Design review of the part shown in the three views and the two pictorial views. Dimensions are in mm from the part's minimum x, y and z. A direction names the side the tool comes from. Give positions to 0.01 mm unless a question says otherwise; leave off trailing zeros. Order: outer loops, then holes, each group sorted by start corner. A loop starts at its lowest first (then second) coordinate and runs counter-clockwise, first axis right, second up. Notation, with made-up numbers: (11, -29.5) - (20, -29.5) arc R20 cw to (20, 6.5) - close; hole circle Ø8 at (-9, 74). An arc over 180 degrees is marked (long way). Put each result on its own line as item: value.
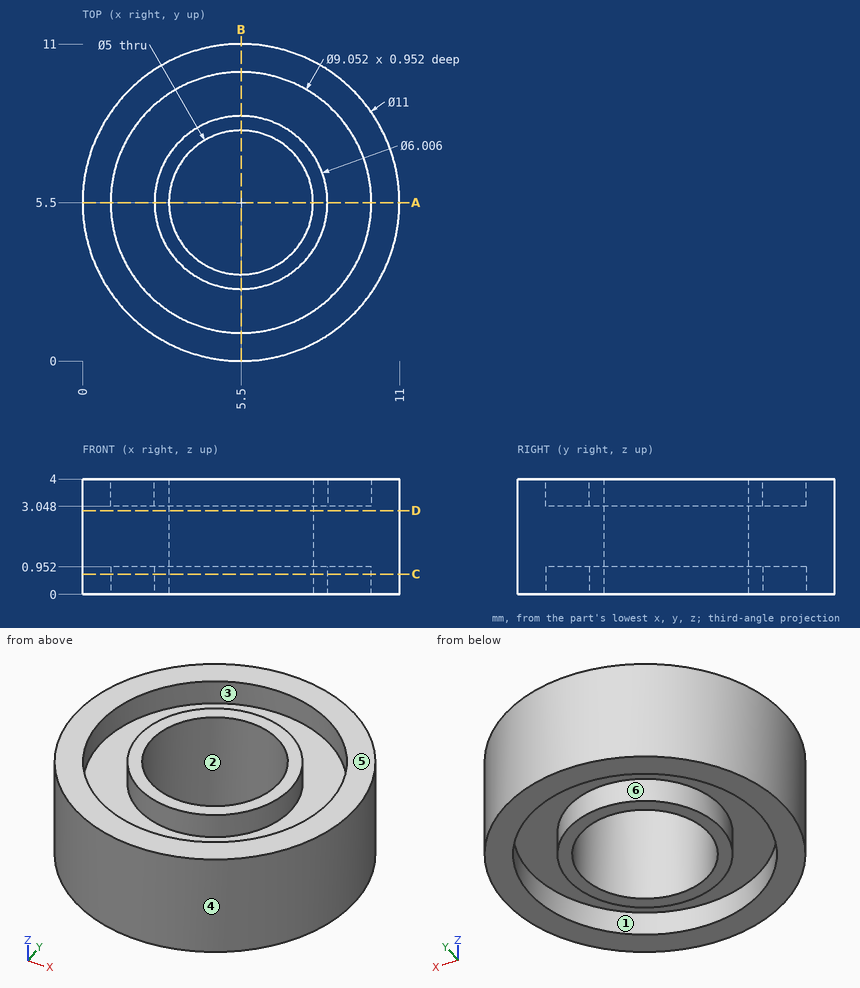
(1) Take a section at A-A, the plane y = 5.5. Write out the cut boundary in (x, z).
The answers:
outline: (0, 0) - (0.97, 0) - (0.97, 0.95) - (2.5, 0.95) - (2.5, 0) - (3, 0) - (3, 4) - (2.5, 4) - (2.5, 3.05) - (0.97, 3.05) - (0.97, 4) - (0, 4) - close; (8, 0) - (8.5, 0) - (8.5, 0.95) - (10.03, 0.95) - (10.03, 0) - (11, 0) - (11, 4) - (10.03, 4) - (10.03, 3.05) - (8.5, 3.05) - (8.5, 4) - (8, 4) - close
(2) The part is to be moulded in two halves that separate along Y. For the marked faces 4, 5 and 6, say which applies: pulls with the +Y half, pulls with the -Y half, needs draft (parallel to the pull), parting line crosses it, or undercut.
The answers:
face 4: parting line crosses it
face 5: needs draft
face 6: undercut
(3) Take a section at D-D, the plane z = 2.9. Write out the cut boundary in (x, y), then the cut area to 3 significant figures.
The answers:
outline: circle Ø11 at (5.5, 5.5); hole circle Ø5 at (5.5, 5.5)
area: 75.4 mm^2
(4) Wall thickness on L1, parallel to Y at x = 5.5, z = 0.45; L2, parallel to Y at x = 5.5, z = 1.75; L3, parallel to Z at x = 4.25, y = 1.75: over which ranges is each line inside the solid? List them lowest first.
The answers:
L1: 0 to 0.97, 2.5 to 3, 8 to 8.5, 10.03 to 11
L2: 0 to 3, 8 to 11
L3: 0.95 to 3.05
(5) For the marked faces 1, 2 and 3, list the 3-axis set-ups (+Z, -Z, +X, -X, +Y, -Y) from which the entire face can be reached by the end or side of a thin tool; tool diameter is ignored.
The answers:
face 1: -Z
face 2: +Z, -Z
face 3: +Z
(6) Take a section at C-C, the plane z = 0.7. Write out the cut boundary in (x, y).
The answers:
outline: circle Ø11 at (5.5, 5.5); circle Ø6.01 at (5.5, 5.5); hole circle Ø9.05 at (5.5, 5.5); hole circle Ø5 at (5.5, 5.5)
